Model file for the job. Use its own axes, mm. A direction names the side the tool comes from. Give positions to 0.01 mm unless a question says otherwise; leave off trailing zeros. Loops run counter-clockwise (first coordinate to the right, second up) from the corner with the lowest first, then second, coordinate; pieces in that order, holes last. Notation, with made-up numbers: M 13,40 L 66,40 A19 cw 66,77 Z; hole C -1.5,88 d5. An arc over 180 degrees is marked long. Use CSV: the item, a comma, the result in double quotes. Start each with the question number.
(1) Slice it at B-B on x = 9.75. List the corners of the cut face in (y, z).
(2) Slice it at C-C on y = 2.15. State how many separate pieces and enclosed holes the cut face has, and give its area (3 significant figures).
(3) Flat gauge pins, fed straight in: P1, Ø1.8, axis at x = 5.5, z = -47, coming from the -Y side; P2, Ø2.5, axis at x = 32.47, z = -32.35, coming from the +Y side. Where does each tip first touch, or does it go through?
(4) Slice it at A-A on z = -40.25. List the corners of the cut face in (x, y), and give its area (3 significant figures).
(5) Two-plate mould, pull along X, no slides. Class faces 3 (the face through (0, 1, -25)), 4 (the face through (50, 1, -25)), 5 (the face through (6.454, 0.74, -47.785)): pulls with the +X half, pulls with the -X half, needs draft (parallel to the pull), parting line crosses it, or undercut.
(6) Wall check: line 1 along Z through (x, y) = (9.75, 0.9); line 2 along X through (y, z) = (0.7, -4); line 3 along X through (y, z) = (0.75, -32.5). Give the ranges that are in metal, low to high. Write a range as from..to.
(7) Slice it at D-D on x = 46.5. List the corners of the cut face in (y, z).
(8) Tool access for faces 1 (the face through (6, 1.5, -5)), 2 (the face through (25, 0, -25)): list every direction of +Z, -Z, +X, -X, +Y, -Y with a clear straight run to the whole face (end or side of a thin tool).
Autodesk Inventor part; units mm, degrees
ref_plane "YZ Plane" through (0, 0, 0) normal (1, 0, 0) x (0, 1, 0)
ref_plane "XZ Plane" through (0, 0, 0) normal (0, 1, 0) x (-1, 0, 0)
ref_plane "XY Plane" through (0, 0, 0) normal (0, 0, 1) x (1, 0, 0)
sketch "Sketch1" plane through (0, 0, 0) normal (0, 1, 0) x (-1, 0, 0)
  circle A0 centre (-17.5282, -17.6529) radius 1.5
  circle A1 centre (-32.4718, -17.6529) radius 1.5
  circle A2 centre (-32.4718, -32.3471) radius 1.5
  circle A3 centre (-40.25, -40.25) radius 1.5
  circle A4 centre (-40.25, -9.75) radius 1.5
  circle A5 centre (-17.5282, -32.3471) radius 1.5
  circle A6 centre (-9.75, -40.25) radius 1.5
  circle A7 centre (-9.75, -9.75) radius 1.5
  line L0 (0, 0) -> (0, -50)
  line L1 (0, -50) -> (-50, -50)
  line L2 (-50, -50) -> (-50, 0)
  line L3 (-50, 0) -> (0, 0)
  circle A8 centre (-4.2426, -4.2426) radius 1.5
  circle A9 centre (-4.2426, -45.7574) radius 1.5
  circle A10 centre (-45.7574, -45.7574) radius 1.5
  circle A11 centre (-45.7574, -4.2426) radius 1.5
  circle A12 centre (-6.6113, -80.0791) radius 3
  circle A13 centre (-15.9332, -80.0791) radius 3
  line L4 (-3.9183, -85.1543) -> (-3.9183, -133.5246) construction
  line L5 (-3.9183, -133.5246) -> (-20.8013, -133.5246) construction
  line L6 (-20.8013, -133.5246) -> (-20.8013, -85.1543) construction
  line L7 (-20.8013, -85.1543) -> (-3.9183, -85.1543) construction
  circle A14 centre (-4.2426, -4.2426) radius 3
  circle A15 centre (-4.2426, -45.7574) radius 3
  circle A16 centre (-45.7574, -45.7574) radius 3
  circle A17 centre (-45.7574, -4.2426) radius 3
  dimension "d2" = 3
  dimension "d3" = 3
  dimension "d4" = 3
  dimension "d5" = 3
  dimension "d6" = 50
  dimension "d7" = 50
  dimension "d12" = 3
  dimension "d13" = 3
  dimension "d14" = 3
  dimension "d15" = 3
  dimension "d16" = 6
  dimension "d17" = 6
  dimension "d21" = 6
  dimension "d22" = 6
  dimension "d23" = 6
  dimension "d24" = 6
extrude "Extrusion1" add sketch "Sketch1" along normal blind 3 contours L0 L1 L2 L3 | A14 | A15 | A16 | A17
fillet "Fillet1" radius 2 4 edges at (0, 1.5, -50) (50, 1.5, -50) (50, 1.5, 0) (0, 1.5, 0)
extrude "Extrusion2" cut sketch "Sketch1" along normal blind 1.5 contours A14 | A15 | A16 | A17
properties part number "Topp 2.1"
Reply:
1,outline,"M 0,-50 L 3,-50 L 3,-41.75 L 0,-41.75 Z; M 0,-38.75 L 3,-38.75 L 3,-11.25 L 0,-11.25 Z; M 0,-8.25 L 3,-8.25 L 3,0 L 0,0 Z"
2,separate pieces,"1"
2,enclosed holes,"12"
2,area,"2,410 mm^2"
3,P1,"stops at y = 1.5"
3,P2,"passes through"
4,outline,"M 0,0 L 8.25,0 L 8.25,3 L 0,3 Z; M 11.25,0 L 38.75,0 L 38.75,3 L 11.25,3 Z; M 41.75,0 L 50,0 L 50,3 L 41.75,3 Z"
4,area,"132 mm^2"
5,face 3,"pulls with the -X half"
5,face 4,"pulls with the +X half"
5,face 5,"undercut"
6,line 1,"z = -50..-41.75, -38.75..-11.25, -8.25..0"
6,line 2,"x = 0..1.25, 7.23..42.77, 48.75..50"
6,line 3,"x = 0..16.04, 19.02..30.98, 33.96..50"
7,outline,"M 0,-50 L 3,-50 L 3,-47.06 L 1.5,-47.06 L 1.5,-48.66 L 0,-48.66 Z; M 0,-42.85 L 1.5,-42.85 L 1.5,-44.45 L 3,-44.45 L 3,-5.55 L 1.5,-5.55 L 1.5,-7.15 L 0,-7.15 Z; M 0,-1.34 L 1.5,-1.34 L 1.5,-2.94 L 3,-2.94 L 3,0 L 0,0 Z"
8,face 1,"-Y"
8,face 2,"+Z, -Z, +X, -X, -Y"
